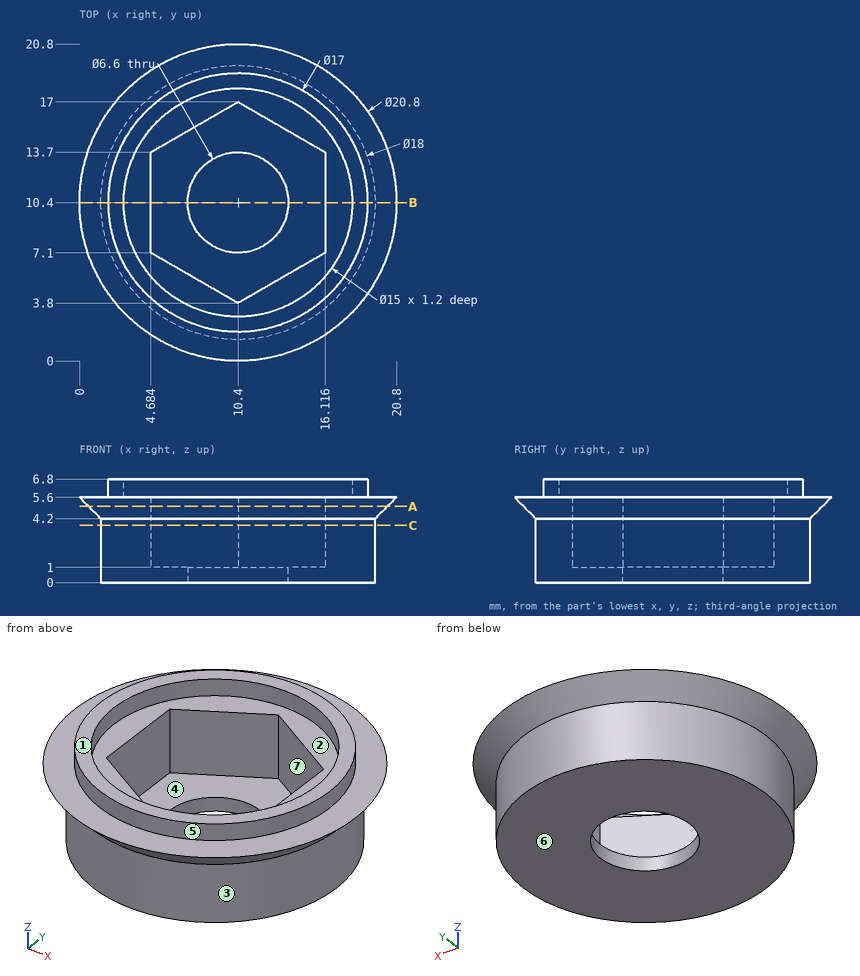
Source: three-view drawing plus pictorial views. Frame: mm from the lowest corner of the part. A direction names the side the tool comes from. Give positions to 0.01 mm unless a question says otherwise; leave off trailing zeros. Write each loop counter-clockwise with the first axis right and the second up, starting at its lowest first coordinate (ties: lowest second). Pieces come first, ordered by that corner, then holes.
(1) Ray query, line 1 (Y direction, x = 10.4, z = 6.05); line 2 (Y direction, x = 10.4, z = 0.4); line 3 (Z direction, x = 8.75, y = 14). Return the intervals inside material, ascending.
(2) Cut plane A-A, the plane z = 5. Return loops of the section in (x, y).
(3) Cut plane C-C, the plane z = 3.75. Return loops of the section in (x, y).
(4) Cut plane B-B, the plane y = 10.4. Return loops of the section in (x, z).
(5) Access query for the marked faces 1, 2 and 3. Directions: +Z, -Z, +X, -X, +Y, -Y. A direction counts if a zero-diameter tool reaches every point of the face in a straight line with its end or side. Return the directions, or none.
(6) Mould query, pull axis X, two halves, no side actions, for the marked faces 4, 5, 6 and 7. Classes: released by +X, released by -X, zero draft, split by the parting line, or undercut.
(7) First-contact query: P1, Ø1, axis at y = 13, z = 4, coming from the -X side; P2, Ø6, axis at x = 10.4, y = 10.4, coming from the +Z side; P3, Ø3, axis at y = 7.5, z = 3.5, coming from the +X side; P4, Ø2, axis at y = 9.5, z = 3.5, coming from the -X side. Flat tips, straight axial feed; report the tip coordinate or a pass-through.
Values follow:
1. line 1: y = 1.9 to 2.9, 17.9 to 18.9
1. line 2: y = 1.4 to 7.1, 13.7 to 19.4
1. line 3: z = 0 to 1
2. outline: circle Ø19.6 at (10.4, 10.4); hole (4.68, 7.1) - (10.4, 3.8) - (16.12, 7.1) - (16.12, 13.7) - (10.4, 17) - (4.68, 13.7) - close
3. outline: circle Ø18 at (10.4, 10.4); hole (4.68, 7.1) - (10.4, 3.8) - (16.12, 7.1) - (16.12, 13.7) - (10.4, 17) - (4.68, 13.7) - close
4. outline: (0, 5.6) - (1.4, 4.2) - (1.4, 0) - (7.1, 0) - (7.1, 1) - (4.68, 1) - (4.68, 5.6) - (2.9, 5.6) - (2.9, 6.8) - (1.9, 6.8) - (1.9, 5.6) - close; (13.7, 0) - (19.4, 0) - (19.4, 4.2) - (20.8, 5.6) - (18.9, 5.6) - (18.9, 6.8) - (17.9, 6.8) - (17.9, 5.6) - (16.12, 5.6) - (16.12, 1) - (13.7, 1) - close
5. face 1: +Z, +X, -X, +Y, -Y
5. face 2: +Z
5. face 3: -Z
6. face 4: undercut
6. face 5: split by the parting line
6. face 6: zero draft
6. face 7: undercut
7. P1: stops at x = 1.45
7. P2: passes through
7. P3: stops at x = 19.82
7. P4: stops at x = 1.14
